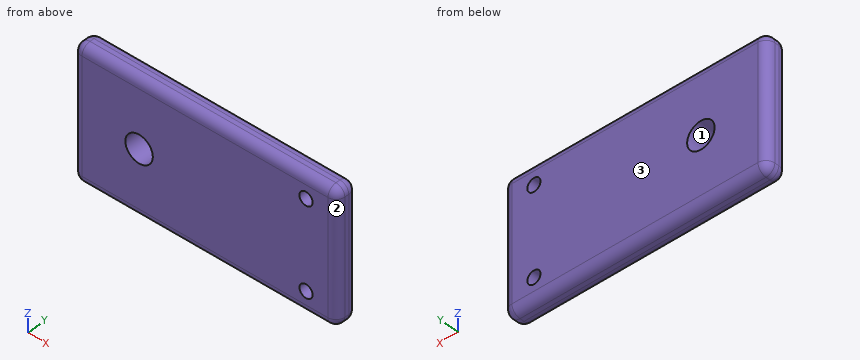
from build123d import *

# Parameters (mm, degrees)
F0_W         = 152.4
F0_H         = 76.2
F0_R         = 7.9375
F1_DEPTH     = 6.35
F2_R         = 5.08
F3_T1_DEPTH  = 2.54
F3_S5_W      = 5.08
F3_S5_H      = 5.08
F3_T6_DEPTH  = 5.08
F3_S11_W     = 5.08
F3_S11_H     = 5.08
F3_T12_DEPTH = 5.08
F4_R         = 3.81
F5_DEPTH     = 25.4


# Not quite as in the source:
# - a fillet or chamfer that OpenCascade refuses, or shapes differently, is made with other operations: its cross-section is extruded or revolved along the edge and cut away or added


with BuildPart() as f1:
    # F0 (on Front) → F1 (new body, symmetric)
    with BuildSketch(Plane.XZ):
        Rectangle(F0_W, F0_H)
        with Locations((-38.1, 0)):
            Circle(F0_R, mode=Mode.SUBTRACT)
    extrude(amount=F1_DEPTH, both=True)

    # F2
    f2_edges = [f1.edges().sort_by_distance(p)[0] for p in [
        (0, -6.35, 38.1),
        (-76.2, -6.35, 0),
        (0, -6.35, -38.1),
        (76.2, -6.35, 0),
        (-76.2, 6.35, 0),
        (-76.2, 0, -38.1),
        (0, 6.35, -38.1),
        (76.2, 6.35, 0),
        (76.2, 0, -38.1),
        (76.2, 0, 38.1),
        (0, 6.35, 38.1),
    ]]
    fillet(f2_edges, radius=F2_R)

    # F3: fillet of radius 5.08 on 1 edges, made by hand

    # F3_s2 → F3_t1 (cut)
    with BuildSketch(Plane.XZ.offset(-1.27)):
        with BuildLine():
            ThreePointArc((-76.2, 33.02), (-74.7121024484, 36.6121024484), (-71.12, 38.1))
            Line((-71.12, 38.1), (-76.2, 38.1))
            Line((-76.2, 38.1), (-76.2, 33.02))
        make_face()
    extrude(amount=F3_T1_DEPTH, mode=Mode.SUBTRACT)


with BuildPart() as f3_tool4:
    # F3_s5 → F3_t6 (new body)
    with BuildSketch(Plane.YZ.offset(-71.12)):
        with Locations((-3.81, 35.56)):
            Rectangle(F3_S5_W, F3_S5_H)
    extrude(amount=-F3_T6_DEPTH)

    # F3_s7 → F3_t8 (revolve, cut)
    with BuildSketch(Plane(origin=(-71.12, -1.27, 33.02), x_dir=(0, 0.7071067812, -0.7071067812), z_dir=(0, 0.7071067812, 0.7071067812))):
        with BuildLine():
            ThreePointArc((0, -5.08), (5.08, 0), (0, 5.08))
            Line((0, 5.08), (0, -5.08))
        make_face()
    revolve(axis=Axis((-71.12, -1.27, 33.02), (-1, 0, 0)), mode=Mode.SUBTRACT)


with BuildPart() as f1_1:
    add(f1.part)

    # F3_t3: cut F3_tool4
    add(f3_tool4.part, mode=Mode.SUBTRACT)


with BuildPart() as f3_tool10:
    # F3_s11 → F3_t12 (new body)
    with BuildSketch(Plane.YZ.offset(-71.12)):
        with Locations((3.81, 35.56)):
            Rectangle(F3_S11_W, F3_S11_H)
    extrude(amount=-F3_T12_DEPTH)

    # F3_s13 → F3_t14 (revolve, cut)
    with BuildSketch(Plane(origin=(-71.12, 1.27, 33.02), x_dir=(0, -0.7071067812, -0.7071067812), z_dir=(0, 0.7071067812, -0.7071067812))):
        with BuildLine():
            ThreePointArc((0, -5.08), (5.08, 0), (0, 5.08))
            Line((0, 5.08), (0, -5.08))
        make_face()
    revolve(axis=Axis((-71.12, 1.27, 33.02), (-1, 0, 0)), mode=Mode.SUBTRACT)


with BuildPart() as f1_2:
    add(f1_1.part)

    # F3_t9: cut F3_tool10
    add(f3_tool10.part, mode=Mode.SUBTRACT)

    # F4 (on face) → F5 (cut)
    with BuildSketch(Plane.XZ.offset(6.35)):
        with Locations((58.42, 25.4)):
            Circle(F4_R)
        with Locations((58.42, -25.4)):
            Circle(F4_R)
    extrude(amount=-F5_DEPTH, mode=Mode.SUBTRACT)


solid = f1_2.part
Check sheet for the modelled part. Datum: model origin and axes. Units: mm. Face numbers are marked on the shaded views. Coordinates: 2 decimals unless noted, no trailing zeros. Loops run counter-clockwise (first coordinate to the right, second up) from the corner with the lowest first, then second, coordinate; pieces in that order, holes last. Notation, with made-up numbers: (61.25, 9.5) -> (65.25, 9.5) arc R27 cw to (65.25, 34.5) -> close; hole circle Ø8 at (-16, -6). An arc over 180 degrees is marked (long way). Write item = value, one per line. Start each with the question number.
1. Draft check along X on the marked faces 1, 2 and 3. Enter one of: released by +X, released by -X, zero draft, split by the parting line, or undercut.
2. Section check A-A on x = 58.42. Record the cut outline in (y, z).
3. Section check B-B on z = 0. Record the cut outline in (x, y), then the cut area to 3 significant figures.
4. Section check C-C on x = -38.1. Record the cut outline in (y, z).
5. Depth check by flat-ended pin: P1, Ø6, axis at x = 6, y = 2.5, coming from the +Z side; P2, Ø7, axis at x = 58.42, z = -25.4, coming from the -Y side; P3, Ø1.5, axis at y = -4, z = -1.5, coming from the +X side; P4, Ø4, axis at y = -3.5, z = -23.5, coming from the +X side. Enter the tip coordinate at first touch or a pass-through.
6. Section check D-D on y = 3. Record the cut outline in (x, z) (1 decimal).
7. Material ranges on line 1 (X direction, y = 1, z = -1); line 2 (Z direction, x = 40, y = -1.5); line 3 (Z direction, x = -38.1, y = -3), recorded low to high.
Responses:
q1.face_1 = undercut
q1.face_2 = released by +X
q1.face_3 = zero draft
q2.outline = (-6.35, -33.02) arc R5.08 ccw to (-1.27, -38.1) -> (1.27, -38.1) arc R5.08 ccw to (6.35, -33.02) -> (6.35, -29.21) -> (-6.35, -29.21) -> close; (-6.35, -21.59) -> (6.35, -21.59) -> (6.35, 21.59) -> (-6.35, 21.59) -> close; (-6.35, 29.21) -> (6.35, 29.21) -> (6.35, 33.02) arc R5.08 ccw to (1.27, 38.1) -> (-1.27, 38.1) arc R5.08 ccw to (-6.35, 33.02) -> close
q3.outline = (-76.2, -1.27) arc R5.08 ccw to (-71.12, -6.35) -> (-46.04, -6.35) -> (-46.04, 6.35) -> (-71.12, 6.35) arc R5.08 ccw to (-76.2, 1.27) -> close; (-30.16, -6.35) -> (71.12, -6.35) arc R5.08 ccw to (76.2, -1.27) -> (76.2, 1.27) arc R5.08 ccw to (71.12, 6.35) -> (-30.16, 6.35) -> close
q3.area = 1,710 mm2
q4.outline = (-6.35, -33.02) arc R5.08 ccw to (-1.27, -38.1) -> (1.27, -38.1) arc R5.08 ccw to (6.35, -33.02) -> (6.35, -7.94) -> (-6.35, -7.94) -> close; (-6.35, 7.94) -> (6.35, 7.94) -> (6.35, 33.02) arc R5.08 ccw to (1.27, 38.1) -> (-1.27, 38.1) arc R5.08 ccw to (-6.35, 33.02) -> close
q5.P1 = 38.1
q5.P2 = through
q5.P3 = 75.8
q5.P4 = 76.19
q6.outline = (-75.9, -33) arc R4.8 ccw to (-71.1, -37.8) -> (71.1, -37.8) arc R4.8 ccw to (75.9, -33) -> (75.9, 33) arc R4.8 ccw to (71.1, 37.8) -> (-71.1, 37.8) arc R4.8 ccw to (-75.9, 33) -> close; hole circle Ø15.9 at (-38.1, 0); hole circle Ø7.6 at (58.4, -25.4); hole circle Ø7.6 at (58.4, 25.4)
q7.line_1 = -76.2 to -45.97, -30.23 to 76.2
q7.line_2 = -38.09 to 38.09
q7.line_3 = -37.8 to -7.94, 7.94 to 37.8
